```python
from build123d import *

# Parameters (mm, degrees)
SKETCH1_R           = 44
BOSS_EXTRUDE1_DEPTH = 3
BOSS_EXTRUDE2_DEPTH = 5
BOSS_EXTRUDE3_DEPTH = 3


with BuildPart() as part:
    # Sketch1 → Boss-Extrude1 (new body)
    with BuildSketch(Plane(origin=(0, 0, 0), x_dir=(1, 0, 0), z_dir=(0, 1, 0))):
        Circle(SKETCH1_R)
    extrude(amount=BOSS_EXTRUDE1_DEPTH)

    # Sketch2 → Boss-Extrude2 (add)
    with BuildSketch(Plane(origin=(0, 3, 0), x_dir=(1, 0, 0), z_dir=(0, 1, 0))):
        with BuildLine():
            Line((-19.168383357, 35.903524611), (-19.921931597, 37.314965382))
            ThreePointArc((-19.921931597, 37.314965382), (4.492861264, -42.060720366), (11.590514748, 40.681076287))
            Line((11.590514748, 40.681076287), (11.152102843, 39.142312172))
            ThreePointArc((11.152102843, 39.142312172), (4.322918521, -40.469771132), (-19.168383357, 35.903524611))
        make_face()
    extrude(amount=BOSS_EXTRUDE2_DEPTH)

    # Sketch3 → Boss-Extrude3 (add)
    with BuildSketch(Plane.XZ):
        with BuildLine():
            Line((-1.173425428, -53.751103926), (-8.173425428, -53.751103926))
            ThreePointArc((-8.173425428, -53.751103926), (-11.001852553, -52.579531051), (-12.173425428, -49.751103926))
            Line((-12.173425428, -49.751103926), (-12.173425428, -33.751103926))
            Line((-12.173425428, -33.751103926), (2.826574572, -33.751103926))
            Line((2.826574572, -33.751103926), (2.826574572, -49.751103926))
            ThreePointArc((2.826574572, -49.751103926), (1.655001697, -52.579531051), (-1.173425428, -53.751103926))
        make_face()
    boss_extrude3 = extrude(amount=-BOSS_EXTRUDE3_DEPTH)

    # Mirror1: Boss-Extrude3 across plane
    add(boss_extrude3.mirror(Plane.XY))


solid = part.part
```
Input: part model. Units: mm. Frame: model coordinates. A direction names the side the tool comes from. Round coordinates to 2 decimals unless told otherwise and drop trailing zeros. Order: outer loops, then holes, each group sorted by start corner. A loop starts at its lowest first (then second) coordinate and runs counter-clockwise, first axis right, second up. Notation, with made-up numbers: (87, 19) - (132, 19) arc R19 cw to (132, 35) - close; hole circle Ø10 at (45.25, 87). An arc over 180 degrees is marked (long way). Answer in a Markdown table with one row per item.
Item 1: Section query D-D (x = -15). Return the cut outline in (y, z), then the cut area to 3 significant figures.
Model answer:
| item | result |
|---|---|
| outline | (0, -41.36) - (3, -41.36) - (3, 37.84) - (8, 37.84) - (8, 39.55) - (3, 39.55) - (3, 41.36) - (0, 41.36) - close |
| area | 257 mm² |
Item 2: Line query: line 1 (X direction, y = 6.1, z = 0); line 2 (Y direction, x = 23, z = 26.5); line 3 (Z direction, x = 0, y = 5.9). Output: solid intervals per line, ascending.
Model answer:
| item | result |
|---|---|
| line 1 | x = -42.3 to -40.7, 40.7 to 42.3 |
| line 2 | y = 0 to 3 |
| line 3 | z = 40.7 to 42.3 |
Item 3: Section query B-B (y = 1.25). Return the cut outline in (x, z), then the cut area to 3 significant figures.
Model answer:
| item | result |
|---|---|
| outline | (-12.17, -49.75) arc R4 ccw to (-8.17, -53.75) - (-1.17, -53.75) arc R4 ccw to (2.83, -49.75) - (2.83, -43.91) arc R44 ccw to (2.83, 43.91) - (2.83, 49.75) arc R4 ccw to (-1.17, 53.75) - (-8.17, 53.75) arc R4 ccw to (-12.17, 49.75) - (-12.17, 42.28) arc R44 ccw to (-12.17, -42.28) - close |
| area | 6,370 mm² |
Item 4: Pin query (flat end, axial travel): pin 1 (3.5 mm diameter, centred on y = 2, z = 46, fed in from +X); pin 2 (3 mm diameter, centred on y = 2, z = -39, fed in from +X); pin 3 (2.5 mm diameter, centred on y = 2, z = 45, fed in from -X). Return the tip coordinate at first contact, or that it passes through.
Model answer:
| item | result |
|---|---|
| pin 1 | stops at x = 2.83 |
| pin 2 | stops at x = 23.02 |
| pin 3 | stops at x = -12.17 |
Item 5: Reachability of faces 1 (the flat face through (2.827, 1, -47)), 2 (the flat face through (-12.173, 1, 46)), 3 (the flat face through (1, 3, -1)) from +Z, -Z, +X, -X, +Y, -Y: full face, straight path, thin tool, end or side. Return the list, or none.
Model answer:
| item | result |
|---|---|
| face 1 | -Z, +X, +Y, -Y |
| face 2 | +Z, -X, +Y, -Y |
| face 3 | +Y |
Item 6: Mould query, pull axis X, two halves, no side actions, for faces 4 (the flat face through (2.827, 1, 47)), 5 (the flat face through (-3, 8, 41)), 6 (the cylindrical face through (5.882, 5.465, 40.273)). Classes: released by +X, released by -X, zero draft, split by the parting line, or undercut.
Model answer:
| item | result |
|---|---|
| face 4 | released by +X |
| face 5 | zero draft |
| face 6 | undercut |
Item 7: Section query A-A (z = 0). Return the cut outline in (x, y), then the cut area to 3 significant figures.
Model answer:
| item | result |
|---|---|
| outline | (-44, 0) - (44, 0) - (44, 3) - (42.3, 3) - (42.3, 8) - (40.7, 8) - (40.7, 3) - (-40.7, 3) - (-40.7, 8) - (-42.3, 8) - (-42.3, 3) - (-44, 3) - close |
| area | 280 mm² |
Item 8: Section query C-C (x = 0). Return the cut outline in (y, z).
Model answer:
| item | result |
|---|---|
| outline | (0, -53.58) - (3, -53.58) - (3, 40.7) - (8, 40.7) - (8, 42.3) - (3, 42.3) - (3, 53.58) - (0, 53.58) - close |
